Could you check a few things on this model? Use its own coordinates, in mm. Round coordinates to 2 decimals unless told otherwise and drop trailing zeros. Order: outer loops, then holes, each group sorted by start corner. A loop starts at its lowest first (then second) coordinate and runs counter-clockwise, first axis right, second up. Notation, with made-up numbers: (34.5, 8) -> (38.5, 8) arc R11 cw to (38.5, 18) -> close; hole circle Ø9 at (-17, 55). An arc over 180 degrees is marked (long way). One line per question, with ' | ' between items.
Autodesk Inventor part; units mm, degrees
ref_plane "YZ Plane" through (0, 0, 0) normal (1, 0, 0) x (0, 1, 0)
ref_plane "XZ Plane" through (0, 0, 0) normal (0, 1, 0) x (-1, 0, 0)
ref_plane "XY Plane" through (0, 0, 0) normal (0, 0, 1) x (1, 0, 0)
sketch "Sketch1" plane through (0, 0, 0) normal (0, 0, 1) x (1, 0, 0)
  line L0 (0, 9.6891) -> (0, -0.0008) construction
  arc A0 (-6.35, -0.0008) -> (6.35, -0.0008) centre (0, -0.0008) ccw
  line L1 (9.3613, -12.4169) -> (3.0751, -6.1307)
  line L2 (5.5891, -3.975) -> (11.6964, -10.0822)
  line L3 (9.3613, -12.4169) -> (12.1811, -14.0872)
  line L4 (12.1811, -14.0872) -> (13.3665, -12.9018)
  line L5 (13.3665, -12.9018) -> (11.6964, -10.0822)
  line L6 (19.3321, -0.0008) -> (-6.0679, -0.0008) construction
  arc A1 (-3.0752, -6.1307) -> (3.0751, -6.1307) centre (0, -0.0008) ccw
  arc A2 (0.9808, -6.7883) -> (3.0751, -6.1307) centre (0, -0.0008) ccw
  arc A3 (-6.8102, -0.809) -> (-5.5892, -3.975) centre (0, -0.0008) ccw
  arc A4 (5.5891, -3.975) -> (6.6548, -1.6576) centre (0, -0.0008) ccw
  arc A5 (5.5891, -3.975) -> (6.6548, -1.6576) centre (0, -0.0008) ccw
  line L7 (5.5891, -3.975) -> (21.5654, -3.975) construction
  line L8 (-9.3614, -12.4169) -> (-3.0752, -6.1307)
  line L9 (-5.5892, -3.975) -> (-11.6964, -10.0822)
  line L10 (-9.3614, -12.4169) -> (-12.1812, -14.0872)
  line L11 (-12.1812, -14.0872) -> (-13.3666, -12.9018)
  line L12 (-13.3666, -12.9018) -> (-11.6964, -10.0822)
  line L13 (9.5758, 1.6559) -> (12.7495, 0.8434)
  line L14 (6.6548, 1.6559) -> (9.5758, 1.6559)
  line L15 (9.5758, -1.6576) -> (12.7495, -0.8451)
  line L16 (6.6548, -1.6576) -> (9.5758, -1.6576)
  circle A6 centre (7.9375, -0.7946) radius 0.254
  circle A7 centre (7.9375, 0.7929) radius 0.254
  circle A8 centre (-5.4113, -6.1454) radius 0.508
  line L17 (12.7495, 0.8434) -> (12.7495, -0.8451)
  circle A9 centre (5.4113, -6.1454) radius 0.508
  line L18 (-2.5412, 6.3492) -> (2.5411, 6.3492)
  line L19 (2.5411, 6.3492) -> (6.35, -0.0008)
  line L20 (5.9486, 1.6559) -> (6.6548, 1.6559)
  line L21 (5.9486, 1.6559) -> (2.8288, 6.8572)
  line L22 (2.8288, 6.8572) -> (-2.8289, 6.8572)
  arc A10 (-6.8565, 0.1423) -> (-5.5892, -3.975) centre (0, -0.0008) ccw
  line L23 (0, 6.3492) -> (-2.5412, 6.3492)
  line L24 (-2.5412, 6.3492) -> (-6.35, -0.0008)
  line L25 (-6.8565, 0.1423) -> (-2.8289, 6.8572)
  line L26 (-2.8289, 6.8572) -> (0, 6.8572)
  point P0 (13.4194, -0.6736)
  point P1 (13.4673, -0.0008)
  point P2 (0, 7.922)
  dimension "GapSize" = 3.048
  dimension "d35" = 12.7
  dimension "d72" = 8.89
  dimension "d73" = 3.2774
  dimension "d77" = 194.36
  dimension "d78" = 1.6764
  dimension "d115" = 90
  dimension "d127" = 0.508
  dimension "d128" = 165.64
  dimension "d154" = 3.302
  dimension "d160" = 3.276
  dimension "d166" = 0.508
  dimension "d168" = 7.9375
  dimension "d169" = 0.863
  dimension "d176" = 1.016
  dimension "d182" = 3.3135
  dimension "d184" = 1.6885
  dimension "d191" = 2.921
  dimension "d234" = 24.3623
  dimension "d238" = 0.508
  dimension "d239" = 0.508
  dimension "d240" = 0.508
  dimension "d241" = 25.4
  dimension "d242" = 0.508
extrude "Extrusion9" add sketch "Sketch1" along normal blind 1.27
fillet "Fillet67" radius 0.254 1 edges at (12.7495, 0.8434, 0.635)
fillet "Fillet68" radius 0.254 1 edges at (12.7495, -0.8451, 0.635)
fillet "Fillet69" radius 1.27 1 edges at (6.35, -0.0008, 0.635)
fillet "Fillet70" radius 1.27 1 edges at (2.8288, 6.8572, 0.635)
fillet "Fillet71" radius 1.27 1 edges at (-2.8289, 6.8572, 0.635)
fillet "Fillet72" radius 1.27 1 edges at (-6.8565, 0.1423, 0.635)
fillet "Fillet73" radius 1.27 1 edges at (-6.35, -0.0008, 0.635)
fillet "Fillet74" radius 1.27 1 edges at (2.5411, 6.3492, 0.635)
fillet "Fillet75" radius 1.27 1 edges at (-2.5412, 6.3492, 0.635)
fillet "Fillet76" radius 0.254 1 edges at (13.3665, -12.9018, 0.635)
fillet "Fillet77" radius 0.254 1 edges at (12.1811, -14.0872, 0.635)
fillet "Fillet78" radius 0.254 1 edges at (-12.1812, -14.0872, 0.635)
fillet "Fillet79" radius 0.254 1 edges at (-13.3666, -12.9018, 0.635)
equation "\"GapSize\" = Thickness"
equation "\"BendRadius\" = Thickness"
equation "\"BendReliefWidth\" = Thickness"
equation "\"BendReliefDepth\" = 0.5 * Thickness"
equation "\"CornerReliefSize\" = 4 * Thickness"
equation "\"MinimumRemnant\" = 2 * Thickness"
equation "\"TransitionRadius\" = BendRadius"
equation "\"JacobiRadiusSize\" = BendRadius"
properties part number "PearHeadbar"
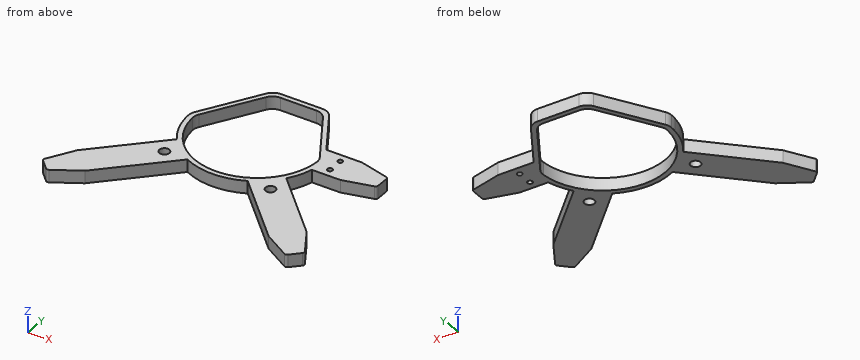
1. I'm going to push flat-ended pins straight in: pin 1 (0.6 mm diameter, centred on y = 0, z = 1, fed in from +X); pin 2 (0.6 mm diameter, centred on x = 8, z = 1, fed in from -Y). Where does each tip first touch, or does it pass through?
From the geometry:
pin 1: stops at x = 12.75 | pin 2: stops at y = -11.36
2. I want a section at C-C on z = 0.4. Count the separate pieces of the cut face and the enclosed holes in it, and give its area (3 significant figures).
From the geometry:
separate pieces: 1 | enclosed holes: 5 | area: 110 mm²
3. I need wall thicknesses on probe 1 along X at (y, z) = (-5.75, 0.65); probe 2 along Y at (x, z) = (5.5, 0.7); probe 3 along X at (y, z) = (-5, 0.8). Which ranges of each line are inside material? Lowest first, please.
From the geometry:
probe 1: x = -7.36 to -5.73, -5.09 to -2.7, 2.7 to 5.09, 5.73 to 7.36 | probe 2: y = -8.56 to -6.65, -5.65 to -3.17, 1.42 to 2.4 | probe 3: x = -6.61 to -3.92, 3.92 to 6.61
4. I want a section at B-B on y = 3.5. List the corners of the cut face in (x, z) for me.
From the geometry:
outline: (-4.84, 0) -> (-4.25, 0) -> (-4.25, 1.27) -> (-4.84, 1.27) -> close; (4.25, 0) -> (4.84, 0) -> (4.84, 1.27) -> (4.25, 1.27) -> close
5. I want a section at A-A on x = 0. List the corners of the cut face in (y, z) for me, and give its area (3 significant figures).
From the geometry:
outline: (-6.86, 0) -> (-6.35, 0) -> (-6.35, 1.27) -> (-6.86, 1.27) -> close; (6.35, 0) -> (6.86, 0) -> (6.86, 1.27) -> (6.35, 1.27) -> close | area: 1.29 mm²
6. I want a section at D-D on x = -10.75. List the corners of the cut face in (y, z) for me, and give its area (3 significant figures).
From the geometry:
outline: (-13.24, 0) -> (-9.14, 0) -> (-9.14, 1.27) -> (-13.24, 1.27) -> close | area: 5.21 mm²
